Geometry: final body of the model. Coordinates: model frame, mm. Give positions to 0.01 mm unless a question says otherwise; leave off trailing zeros. Loops run counter-clockwise (first coordinate to the right, second up) from the corner with the lowest first, then second, coordinate; pieces in that order, holes last. Notation, with made-up numbers: (85, 88) -> (143, 88) arc R10 cw to (143, 106) -> close; hole circle Ø4 at (55, 29.25). An arc over 180 degrees is marked (long way). One line per question, with ' | ' between items. Start each with the question number.
Item 1: Section B-B on y = -0.85. Give the number of separate pieces and of enclosed holes in the cut face, then the cut area to 3 significant figures.
Item 2: Pin query (flat end, axial travel): P1, Ø1.5, axis at y = -0.5, z = -7.5, coming from the +X side; P2, Ø4, axis at x = 0, z = 12.75, coming from the -Y side. Return the tip coordinate at first contact, or that it passes through.
Item 3: Section A-A on x = 0. Return loops of the section in (y, z).
Item 4: Material intervals for line 1 along Z through (x, y) = (-1, -0.2); line 2 along X through (y, z) = (-1.9, 9.5); line 3 along Z through (x, y) = (-9, -1.9), sorted ascending. Write a range as [from, to].
from build123d import *

# Parameters (mm, degrees)
F0_R     = 17.5
F0_R_2   = 2.5
F0_R_3   = 1.25
F1_DEPTH = 2.5


# Not quite as in the source:
# - the program builds the solid bodies; features that only make, move or delete a surface that nothing else refers to are left out


with BuildPart() as f1:
    # F0 (on Front) → F1 (new body)
    with BuildSketch(Plane.XZ):
        Circle(F0_R)
        with BuildLine():
            ThreePointArc((1.4972975656, -12.41), (1.4993242392, -12.454979718), (1.5, -12.5))
            ThreePointArc((1.5, -12.5), (-0.045020282, -13.9993242392), (-1.4972975656, -12.41))
            ThreePointArc((-1.4972975656, -12.41), (-4.9790100681, -11.4655771221), (-8.0460146394, -9.5661720883))
            ThreePointArc((-8.0460146394, -9.5661720883), (-10.3118696418, -9.6536659725), (-10.0753310722, -7.3984933456))
            ThreePointArc((-10.0753310722, -7.3984933456), (-11.6269109472, -4.5896559594), (-12.4122705024, -1.4783575263))
            ThreePointArc((-12.4122705024, -1.4783575263), (-13.658382684, 0), (-12.4122705024, 1.4783575263))
            ThreePointArc((-12.4122705024, 1.4783575263), (-11.6269110451, 4.5896557115), (-10.0753313878, 7.3984929159))
            ThreePointArc((-10.0753313878, 7.3984929159), (-10.3118706248, 9.6536659173), (-8.0460151958, 9.5661716203))
            ThreePointArc((-8.0460151958, 9.5661716203), (-4.9630114991, 11.472511358), (-1.4626687852, 12.4141290482))
            ThreePointArc((-1.4626687852, 12.4141290482), (-0.167324239, 14.2373289873), (1.5000009313, 12.7466907725))
            ThreePointArc((1.5000009313, 12.7466907725), (1.4906391339, 12.5793654932), (1.4626705992, 12.4141288344))
            ThreePointArc((1.4626705992, 12.4141288344), (4.2850452641, 11.7425886024), (6.8765961266, 10.4385068718))
            ThreePointArc((6.8765961266, 10.4385068718), (8.5606760335, 11.2696593384), (9.736322552, 9.8051475361))
            ThreePointArc((9.736322552, 9.8051475361), (9.5663280132, 9.1115442827), (9.0948752545, 8.5751527162))
            ThreePointArc((9.0948752545, 8.5751527162), (11.2789515194, 5.388436937), (12.3856373166, 1.6870057091))
            ThreePointArc((12.3856373166, 1.6870057091), (13.5512317227, 1.3135614646), (14.0505886972, 0.1961029484))
            ThreePointArc((14.0505886972, 0.1961029484), (13.5685677546, -0.9055860452), (12.4322971789, -1.2992254827))
            ThreePointArc((12.4322971789, -1.2992254827), (11.6124376907, -4.6261529244), (9.9200203194, -7.6054715083))
            ThreePointArc((9.9200203194, -7.6054715083), (10.3020717987, -8.1159348628), (10.4375838551, -8.7389698954))
            ThreePointArc((10.4375838551, -8.7389698954), (9.4776271369, -10.1383816482), (7.8264461833, -9.7466271161))
            ThreePointArc((7.8264461833, -9.7466271161), (4.8483438568, -11.5214392263), (1.4972975656, -12.41))
        make_face(mode=Mode.SUBTRACT)
        with BuildLine():
            ThreePointArc((-1.4972975656, -12.41), (0, -11), (1.4972975656, -12.41))
            ThreePointArc((1.4972975656, -12.41), (4.8483438568, -11.5214392263), (7.8264461833, -9.7466271161))
            ThreePointArc((7.8264461833, -9.7466271161), (7.8650737925, -7.690293508), (9.9200203194, -7.6054715083))
            ThreePointArc((9.9200203194, -7.6054715083), (11.6124376907, -4.6261529244), (12.4322971789, -1.2992254827))
            ThreePointArc((12.4322971789, -1.2992254827), (11.0507717691, 0.1726683089), (12.3856373166, 1.6870057091))
            ThreePointArc((12.3856373166, 1.6870057091), (11.2789515194, 5.388436937), (9.0948752545, 8.5751527162))
            ThreePointArc((9.0948752545, 8.5751527162), (7.271534517, 8.6565901594), (6.8765961266, 10.4385068718))
            ThreePointArc((6.8765961266, 10.4385068718), (4.2850452641, 11.7425886024), (1.4626705992, 12.4141288344))
            ThreePointArc((1.4626705992, 12.4141288344), (8.217e-07, 11.2466907725), (-1.4626687852, 12.4141290482))
            ThreePointArc((-1.4626687852, 12.4141290482), (-4.9630114991, 11.472511358), (-8.0460151958, 9.5661716203))
            ThreePointArc((-8.0460151958, 9.5661716203), (-7.8015231838, 9.1254022263), (-7.7168385163, 8.6285294965))
            ThreePointArc((-7.7168385163, 8.6285294965), (-8.5232029157, 7.298540905), (-10.0753313878, 7.3984929159))
            ThreePointArc((-10.0753313878, 7.3984929159), (-11.6269110451, 4.5896557115), (-12.4122705024, 1.4783575263))
            ThreePointArc((-12.4122705024, 1.4783575263), (-11.1916437657, 1.146915805), (-10.658382684, 0))
            ThreePointArc((-10.658382684, 0), (-11.1916437657, -1.146915805), (-12.4122705024, -1.4783575263))
            ThreePointArc((-12.4122705024, -1.4783575263), (-11.6269109472, -4.5896559594), (-10.0753310722, -7.3984933456))
            ThreePointArc((-10.0753310722, -7.3984933456), (-8.5232023173, -7.2985407313), (-7.716837585, -8.6285294965))
            ThreePointArc((-7.716837585, -8.6285294965), (-7.8015223518, -9.1254025092), (-8.0460146394, -9.5661720883))
            ThreePointArc((-8.0460146394, -9.5661720883), (-4.9790100681, -11.4655771221), (-1.4972975656, -12.41))
        make_face()
        Circle(F0_R_2, mode=Mode.SUBTRACT)
        Circle(F0_R_2)
        Circle(F0_R_3, mode=Mode.SUBTRACT)
    extrude(amount=F1_DEPTH)


solid = f1.part
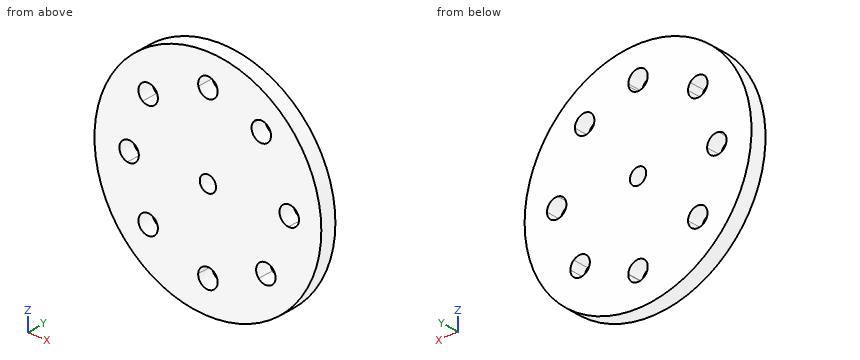
Result sheet:
1) separate pieces: 1 | enclosed holes: 9 | area: 901 mm²
2) P1: stops at x = 16.15 | P2: stops at y = -2.5
3) outline: (-2.5, -17.5) -> (0, -17.5) -> (0, -14) -> (-2.5, -14) -> close; (-2.5, -11) -> (0, -11) -> (0, -1.25) -> (-2.5, -1.25) -> close; (-2.5, 1.25) -> (0, 1.25) -> (0, 11.25) -> (-2.5, 11.25) -> close; (-2.5, 14.25) -> (0, 14.25) -> (0, 17.5) -> (-2.5, 17.5) -> close
4) line 1: z = [-17.47, -13.62], [-11.38, -0.75], [0.75, 11.63], [13.86, 17.47] | line 2: x = [-14.7, -10.44], [-8, 6.77], [9.7, 14.7] | line 3: z = [-15.01, -10.11], [-7.14, 7.14], [10.11, 15.01]
